Can you work these out from the drawing? Everything is in mm from the part's minimum corner. Coordinates: 2 decimals unless noted, no trailing zeros. Loops run counter-clockwise (first coordinate to the right, second up) from the corner with the lowest first, then second, coordinate; pieces in that order, holes last. Notation, with made-up numbers: M 7.5,-16.75 L 43.5,-16.75 A22 cw 43.5,-7.75 Z; hole C -16,20.25 d9. An arc over 180 degrees is marked long. Use CSV: the item, a comma, the result in double quotes. Start each with the question number.
Q1. If we section it at A-A (x = 55): Please give me the cut outline in (y, z).
Q2. For pin 1 Ø1.3 at (y, z) = (8, 2) entering from +X; pin 2 Ø0.5 at (y, z) = (20.5, 2) entering from +X; pin 3 Ø0.6 at (x, y) = (28, 15) entering from +Z, each with a flat end and sliding along its axis, tell me the tip position at first contact or that it passes through.
Q3. If we section it at B-B (y = 8.2): Please give me the cut outline in (x, z), and give its area (3 significant figures).
Q4. Please list where these lines run through material, in increasing order: probe 1 along Y at (x, z) = (44, 3.05); probe 2 along Y at (x, z) = (73.75, 1.6); probe 3 along Z at (x, y) = (7, 41). Write a range as [from, to].
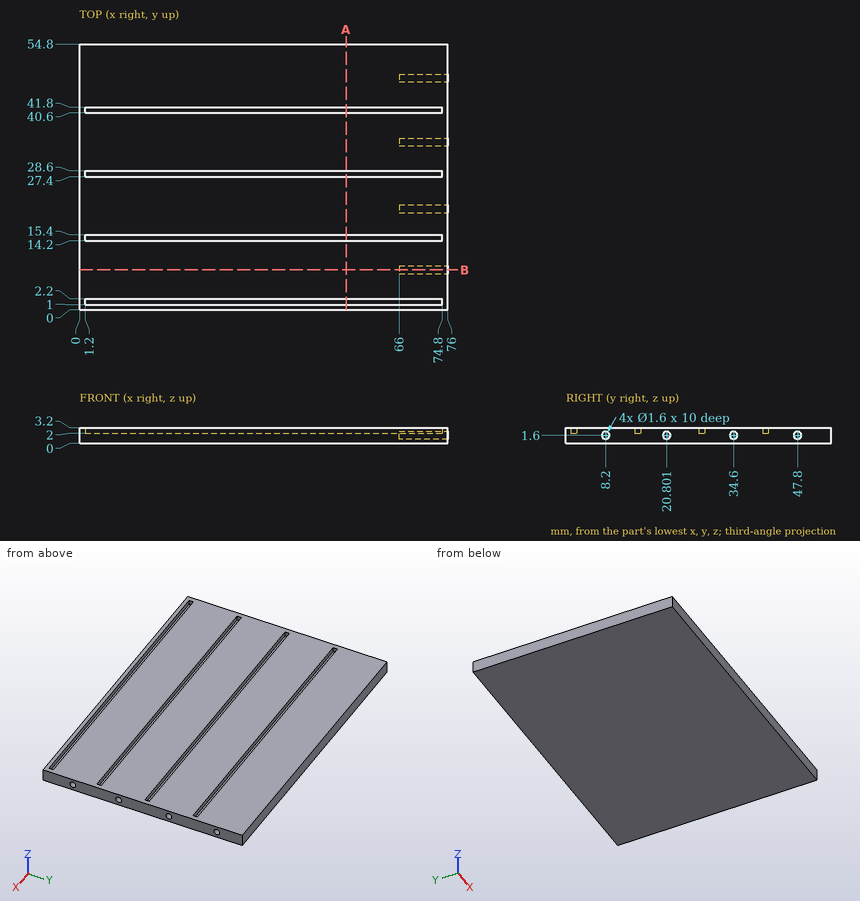
Results below:
1,outline,"M 0,0 L 54.8,0 L 54.8,3.2 L 41.8,3.2 L 41.8,2 L 40.6,2 L 40.6,3.2 L 28.6,3.2 L 28.6,2 L 27.4,2 L 27.4,3.2 L 15.4,3.2 L 15.4,2 L 14.2,2 L 14.2,3.2 L 2.2,3.2 L 2.2,2 L 1,2 L 1,3.2 L 0,3.2 Z"
2,pin 1,"x = 76"
2,pin 2,"x = 66"
2,pin 3,"z = 2"
3,outline,"M 0,0 L 76,0 L 76,0.8 L 66,0.8 L 66,2.4 L 76,2.4 L 76,3.2 L 0,3.2 Z"
3,area,"227 mm^2"
4,probe 1,"[0, 1], [2.2, 14.2], [15.4, 27.4], [28.6, 40.6], [41.8, 54.8]"
4,probe 2,"[0, 7.4], [9, 20], [21.6, 33.8], [35.4, 47], [48.6, 54.8]"
4,probe 3,"[0, 2]"
